Part model, mm, in its own coordinate system. A direction names the side the tool comes from. Round coordinates to 2 decimals unless told otherwise and drop trailing zeros. Loops run counter-clockwise (first coordinate to the right, second up) from the corner with the lowest first, then second, coordinate; pieces in that order, holes last.
(1) Cut at D-D on x = -27. List the corners of the cut face in (y, z) (3 decimals).
(2) Flat gauge pin, fed straight in: pin 1 (1 mm diameter, centred on x = 1.5, y = -2.5, fed in from +Z) (3 decimals). Where does the tip first touch, or does it go through?
(3) Mould opens along X. For faces 3 (the face through (0.58, -0.42, 3.53)), 4 (the face through (-13, -2, -14.978)), 5 (the face through (-26.295, -0.655, 3.528)), 6 (the face through (-31.504, -2.022, -14.214)) say: +X half, -X half, draft (parallel to the pull), parting line (faces both ways), or undercut.
(4) Cut at B-B on y = -1.4. List the corners of the cut face in (x, z) (1 decimal), then the cut area to 3 significant figures.
(5) Probe probe 1 along X at (y, z) = (-1.65, 6.5); probe 2 along X at (y, z) = (-2.55, -1.5); probe 3 along X at (y, z) = (-0.35, 8). List the from-to ranges inside material, lowest first.
(6) Tool access for faces 1 (the face through (-13, -2, 10.422)), 2 (the face through (-27, -2, -3.175)): list every direction of +Z, -Z, +X, -X, +Y, -Y with a clear straight run to the whole face (end or side of a thin tool).
(7) Cut at C-C on z = 5.5. List the corners of the cut face in (x, y) (1 decimal).
(8) Cut at A-A on x = 1. List the corners of the cut face in (y, z) (3 decimals), then the cut area to 3 significant figures.
from build123d import *

# Parameters (mm, degrees)
F0_W          = 38.1
F0_H          = 25.4
F1_DEPTH      = 3.9878
F2_R          = 2.54
F3_R          = 2.54
F4_R          = 2.54
F5_R          = 2.54
F6_R          = 1.5875
F7_DEPTH      = 10.421824
F7_DEPTH_BACK = 3.175


with BuildPart() as f1:
    # F0 (on Front) → F1 (new body)
    with BuildSketch(Plane.XZ):
        with Locations((-13.178508, -2.278176)):
            Rectangle(F0_W, F0_H)
    extrude(amount=F1_DEPTH)

    # F2
    f2_edges = [f1.edges().sort_by_distance(p)[0] for p in [
        (-32.228508, -1.9939, -14.978176),
    ]]
    fillet(f2_edges, radius=F2_R)

    # F3
    f3_edges = [f1.edges().sort_by_distance(p)[0] for p in [
        (5.871492, -1.9939, -14.978176),
    ]]
    fillet(f3_edges, radius=F3_R)

    # F4
    f4_edges = [f1.edges().sort_by_distance(p)[0] for p in [
        (-32.228508, -1.9939, 10.421824),
    ]]
    fillet(f4_edges, radius=F4_R)

    # F5
    f5_edges = [f1.edges().sort_by_distance(p)[0] for p in [
        (5.871492, -1.9939, 10.421824),
    ]]
    fillet(f5_edges, radius=F5_R)

    # F6 (on Top) → F7 (cut, two sides)
    with BuildSketch(Plane.XY) as f7_sk:
        with Locations((-27.148508, -1.9939)):
            Circle(F6_R)
        with Locations((0.791492, -1.9939)):
            Circle(F6_R)
    extrude(amount=F7_DEPTH, mode=Mode.SUBTRACT)
    extrude(f7_sk.sketch, amount=-F7_DEPTH_BACK, mode=Mode.SUBTRACT)


solid = f1.part
Final values:
1. outline: (-3.988, -14.978) - (0, -14.978) - (0, 10.422) - (-0.413, 10.422) - (-0.413, -3.175) - (-3.574, -3.175) - (-3.574, 10.422) - (-3.988, 10.422) - close
2. pin 1: stops at z = -3.175
3. face 3: undercut
3. face 4: draft
3. face 5: undercut
3. face 6: -X half
4. outline: (-32.2, -12.4) arc R2.5 ccw to (-29.7, -15) - (3.3, -15) arc R2.5 ccw to (5.9, -12.4) - (5.9, 7.9) arc R2.5 ccw to (3.3, 10.4) - (2.3, 10.4) - (2.3, -3.2) - (-0.7, -3.2) - (-0.7, 10.4) - (-25.7, 10.4) - (-25.7, -3.2) - (-28.6, -3.2) - (-28.6, 10.4) - (-29.7, 10.4) arc R2.5 ccw to (-32.2, 7.9) - close
4. area: 882 mm2
5. probe 1: x = -32.23 to -28.7, -25.6 to -0.76, 2.34 to 5.87
5. probe 2: x = -32.23 to -28.64, -25.66 to -0.7, 2.28 to 5.87
5. probe 3: x = -32.23 to 5.87
6. face 1: +Z, +X, -X, +Y, -Y
6. face 2: +Z
7. outline: (-32.2, -4) - (5.9, -4) - (5.9, 0) - (-32.2, 0) - close; hole circle Ø3.2 at (-27.1, -2); hole circle Ø3.2 at (0.8, -2)
8. outline: (-3.988, -14.978) - (0, -14.978) - (0, 10.422) - (-0.42, 10.422) - (-0.42, -3.175) - (-3.568, -3.175) - (-3.568, 10.422) - (-3.988, 10.422) - close
8. area: 58.5 mm2
